Geometry: final body of the model. Coordinates: model frame, mm. A direction names the side the tool comes from. Round coordinates to 2 decimals unless told otherwise and drop trailing zeros. Loops run counter-clockwise (first coordinate to the right, second up) from the corner with the lowest first, then second, coordinate; pieces in that order, holes last. Notation, with made-up numbers: (49.25, 68.25) - (69.25, 68.25) arc R18 cw to (69.25, 88.25) - close; hole circle Ø8 at (-3, 2.25). An arc over 180 degrees is marked (long way). Use CSV: the item, a comma, the result in double quotes.
from build123d import *

# Parameters (mm, degrees)
ESBO_O1_W                = 55
ESBO_O1_H                = 55
RESSALTO_EXTRUS_O1_DEPTH = 2
ESBO_O3_W                = 55
ESBO_O3_H                = 55
ESBO_O3_R                = 25
RESSALTO_EXTRUS_O3_DEPTH = 0.5


with BuildPart() as part:
    # Esboço1 → Ressalto-extrusão1 (new body)
    with BuildSketch(Plane(origin=(0, 0, 0), x_dir=(1, 0, 0), z_dir=(0, 1, 0))):
        Rectangle(ESBO_O1_W, ESBO_O1_H)
    extrude(amount=RESSALTO_EXTRUS_O1_DEPTH)

    # Esboço3 → Ressalto-extrusão3 (add)
    with BuildSketch(Plane.XZ):
        Rectangle(ESBO_O3_W, ESBO_O3_H)
        with Locations(Location((0, 0, 0), (0, 0, 270))):
            Circle(ESBO_O3_R, mode=Mode.SUBTRACT)
    extrude(amount=RESSALTO_EXTRUS_O3_DEPTH)


solid = part.part
Item 1: Pin query (flat end, axial travel): P1, Ø5, axis at x = -20.5, z = 2.5, coming from the -Y side. Return the tip coordinate at first contact, or that it passes through.
Final values:
P1,"stops at y = 0"
Item 2: Mould query, pull axis X, two halves, no side actions, for faces 1 (the flat face through (0, 1, -27.5)), 2 (the flat face through (-27.5, 1, 0)), 3 (the flat face through (27.5, 1, 0)), 4 (the flat face through (0, 0, 0)). Classes: released by +X, released by -X, zero draft, split by the parting line, or undercut.
Final values:
face 1,"zero draft"
face 2,"released by -X"
face 3,"released by +X"
face 4,"undercut"
Item 3: Reachability of faces 5 (the cylindrical face through (7.509, -0.246, -23.846)), 6 (the flat face through (0, 2, 0)) from +Z, -Z, +X, -X, +Y, -Y: full face, straight path, thin tool, end or side. Return the list, or none.
Final values:
face 5,"-Y"
face 6,"+Z, -Z, +X, -X, +Y"
Item 4: Section B-B on x = 0. Return the cut outline in (y, z), plus the area to 4 significant figures.
Final values:
outline,"(-0.5, -27.5) - (2, -27.5) - (2, 27.5) - (-0.5, 27.5) - (-0.5, 25) - (0, 25) - (0, -25) - (-0.5, -25) - close"
area,"112.5 mm²"
Item 5: Section A-A on z = 0. Return the cut outline in (x, y).
Final values:
outline,"(-27.5, -0.5) - (-25, -0.5) - (-25, 0) - (25, 0) - (25, -0.5) - (27.5, -0.5) - (27.5, 2) - (-27.5, 2) - close"
Item 6: Material intervals for line 1 (X direction, y = -0.3, z = 0); line 2 (Y direction, x = 5, z = -3); line 3 (Z direction, x = -12, y = -0.4), sorted ascending.
Final values:
line 1,"x = -27.5 to -25, 25 to 27.5"
line 2,"y = 0 to 2"
line 3,"z = -27.5 to -21.93, 21.93 to 27.5"
